Here's how the part is built. I have some questions about the finished solid (model axes, mm). Face numbers are marked on the shaded views. A direction names the side the tool comes from. Coordinates: 2 decimals unless noted, no trailing zeros. Write each loop counter-clockwise with the first axis right and the second up, starting at its lowest first coordinate (ties: lowest second). Pieces come first, ordered by that corner, then holes. Notation, with made-up numbers: (23.5, 2.25) -> (27.5, 2.25) arc R21 ccw to (27.5, 20.25) -> close; hole circle Ø4 at (32, 80). An arc over 180 degrees is marked (long way). Use a Markdown table: item, result. Add a question column.
Autodesk Inventor part; units mm, degrees
ref_plane "YZ Plane" through (0, 0, 0) normal (1, 0, 0) x (0, 1, 0)
ref_plane "XZ Plane" through (0, 0, 0) normal (0, 1, 0) x (-1, 0, 0)
ref_plane "XY Plane" through (0, 0, 0) normal (0, 0, 1) x (1, 0, 0)
sketch "草图1" plane through (0, 0, 0) normal (0, 0, 1) x (1, 0, 0)
  circle A0 centre (0, 0) radius 1.65
  circle A1 centre (0, 0) radius 0.55 construction
  line L0 (0, 1.65) -> (0, 1.35)
  line L1 (0, 1.35) -> (0.2766, 1.6266)
  line L2 (0, 1.35) -> (-0.2766, 1.6266)
  line L3 (0, 1.35) -> (0.3912, 1.35) construction
  line L4 (0, 0) -> (0, 1.65) construction
  line L5 (0, 0) -> (-1.65, 0) construction
  line L6 (0, 0) -> (0, -1.65) construction
  circle A2 centre (0, 0.55) radius 0.15
  circle A3 centre (0, -0.55) radius 0.15
  circle A4 centre (-0.55, 0) radius 0.15
  circle A5 centre (-0.55, 0) radius 0.4
  line L7 (0, -1.65) -> (0, -1.35)
  line L8 (0, -1.35) -> (0.2766, -1.6266)
  line L9 (0, -1.35) -> (-0.2766, -1.6266)
  line L10 (0, -1.35) -> (0.3912, -1.35) construction
  line L11 (-1.35, 0) -> (-1.35, 0.5)
  line L12 (-1.35, 0.5) -> (-1.5724, 0.5)
  line L13 (-1.35, 0) -> (-1.35, -0.5)
  line L14 (-1.35, -0.5) -> (-1.5724, -0.5)
  point P0 (-0.2766, -1.6266)
  point P1 (0.2766, -1.6266)
  dimension "d0" = 3.3
  dimension "d1" = 1.1
  dimension "d5" = 0.3
  dimension "d6" = 45
  dimension "d7" = 135
  dimension "d8" = 0.3
  dimension "d9" = 0.3
  dimension "d10" = 0.3
  dimension "d11" = 0.8
  dimension "d12" = 0.5
  dimension "d13" = 0.5
  dimension "d14" = 0.3
extrude "拉伸1" add sketch "草图1" along normal blind 1 contours A0 L8 L9 L14 L13 L11 L12 L2 L1 | A2 | A3 | A4 | A5
extrude "拉伸2" add sketch "草图1" against normal blind 5 contours A2 | A3 | A4
extrude "拉伸3" add sketch "草图1" against normal blind 0.3 contours A5
sketch "草图2" plane through (0, 0, 1) normal (0, 0, 1) x (1, 0, 0)
  circle A0 centre (0, 0) radius 1.1
  circle A1 centre (0, 0) radius 1.25
  dimension "d21" = 2.2
  dimension "d22" = 2.5
extrude "拉伸4" add sketch "草图2" along normal blind 2.27 contours A0
extrude "拉伸5" add sketch "草图2" along normal blind 0.3
sketch "草图3" plane through (0, 0, 0) normal (1, 0, 0) x (0, 1, 0)
  line L0 (1.1, 3.27) -> (-1.1, 3.27)
  line L1 (0, 3.27) -> (-0.8, 3.27)
  line L2 (-0.8, 3.27) -> (-0.5879, 3.0579)
  line L3 (-0.5879, 3.0579) -> (0, 3.0579)
  line L4 (0, 3.0579) -> (0, 3.27)
  point P0 (0, 0)
  dimension "d27" = 0.8
  dimension "d28" = 0.3
  dimension "d29" = 45
revolve "旋转1" cut sketch "草图3" angle 360 about axis through (0, 0, 3.0579) along (0, 0, 1)
fillet "圆角1" radius 0.1 2 edges at (-1.1, 0, 3.27) (-1.1, 0, 1.3)
properties part number "CAN_φ3.3" material "黄铜，软黄"
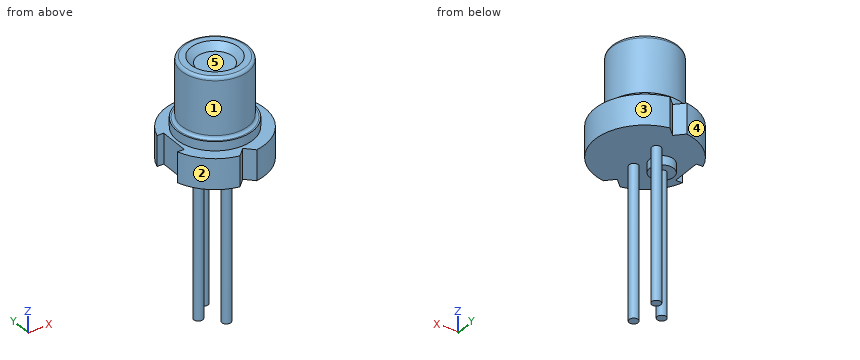
Q1. Suppose I cut it at A-A, the plane y = 0. Write out the boundary of the cut face in (x, z), and give its area (3 significant figures).
Q2. Suppose I cut it at B-B, the plane z = -3.75. Write out the boundary of the cut face in (x, y).
Q3. Which directions (+Z, -Z, +X, -X, +Y, -Y) give clear straight access to the entire face, cutting with the end or side of a thin tool? Please do the marked faces 1 and 2.
Q4. Thinking about a two-plate mould opening in Y: for the marked faces 3, 4 and 5, which applies, released by +Y, released by -Y, zero draft, split by the parting line, or undercut?
Q5. Suppose I cut it at C-C, the plane x = 1.4. Write out the boundary of the cut face in (y, z).
Q6. Please list where these lines run through material, in increasing order: line 1 (Z direction, x = -1.3, y = -0.75); line 2 (Z direction, x = 0.3, y = -0.95); line 3 (Y direction, x = 0.6, z = 0.5).
Q7. Will these pins go through, and if not, where does the flat tip stop? pin 1 (0.8 mm diameter, centred on y = 0, z = 0.5, fed in from -X); pin 2 (0.6 mm diameter, centred on x = 0, y = 0, fed in from +Z); pin 3 (1 mm diameter, centred on x = 1, z = -3, fed in from +Y) (3 decimals).
Answer key:
| question | item | result |
|---|---|---|
| 1 | outline | (-1.35, 0) -> (-0.95, 0) -> (-0.95, -0.3) -> (-0.7, -0.3) -> (-0.7, -5) -> (-0.4, -5) -> (-0.4, -0.3) -> (-0.15, -0.3) -> (-0.15, 0) -> (1.65, 0) -> (1.65, 1) -> (1.25, 1) -> (1.25, 1.3) -> (1.2, 1.3) arc R0.1 cw to (1.1, 1.4) -> (1.1, 3.17) arc R0.1 ccw to (1, 3.27) -> (0.8, 3.27) -> (0.59, 3.06) -> (-0.59, 3.06) -> (-0.8, 3.27) -> (-1, 3.27) arc R0.1 ccw to (-1.1, 3.17) -> (-1.1, 1.4) arc R0.1 cw to (-1.2, 1.3) -> (-1.25, 1.3) -> (-1.25, 1) -> (-1.35, 1) -> close |
| 1 | area | 9.44 mm^2 |
| 2 | outline | circle Ø0.3 at (-0.55, 0); circle Ø0.3 at (0, -0.55); circle Ø0.3 at (0, 0.55) |
| 3 | face 1 | +Z |
| 3 | face 2 | +Z, -Z, -X, -Y |
| 4 | face 3 | split by the parting line |
| 4 | face 4 | released by +Y |
| 4 | face 5 | undercut |
| 5 | outline | (-0.87, 0) -> (0.87, 0) -> (0.87, 1) -> (-0.87, 1) -> close |
| 6 | line 1 | z = 0 to 1 |
| 6 | line 2 | z = 0 to 3.27 |
| 6 | line 3 | y = -1.54 to 1.54 |
| 7 | pin 1 | stops at x = -1.35 |
| 7 | pin 2 | stops at z = 3.06 |
| 7 | pin 3 | passes through |
